Source: CAD feature listing. Evaluate the final solid. Frame: model axes, mm. Face numbers are marked on the shaded views. Coordinates: 2 decimals unless noted, no trailing zeros. Write each loop counter-clockwise with the first axis right and the second up, starting at its lowest first coordinate (ties: lowest second). Pieces come first, ordered by that corner, then holes. Notation, with made-up numbers: M 17.25,-23 L 46.25,-23 A27 cw 46.25,-7 Z; hole C -40,37 d2. An arc over 180 degrees is marked long. Answer as CSV lines item,"result". Start each with the question number.
1. Line query: probe 1 along Y at (x, z) = (14.4, 1.15) (3 decimals); probe 2 along X at (y, z) = (6.35, 0.2); probe 3 along Y at (x, z) = (25, 0.5). Output: solid intervals per line, ascending. Write a range as [from, to].
2. Section A-A on y = 6.35. Return the cut outline in (x, z) (1 decimal), plus the area to 3 significant figures.
3. Section C-C on x = 36.4. Return the cut outline in (y, z) (3 decimals), plus the area to 3 significant figures.
4. Section B-B on x = 25.4. Return the cut outline in (y, z) (3 decimals), plus the area to 3 significant figures.
5. Section D-D on y = 40. Return the cut outline in (x, z) (3 decimals), plus the area to 3 significant figures.
6. Mould query, pull axis X, two halves, no side actions, for the marked faces 1, 2 and 3. Classes: pulls with the +X half, pulls with the -X half, needs draft (parallel to the pull), parting line crosses it, or undercut.
7. Contact query for a flat-ended pin moving along its axis: pin 1 Ø12 at (x, y) = (19.5, 27.5) entering from -Z. Output: stop coordinate, or through.
Solid Edge part; units mm, degrees
sketch "Sketch1" plane through (0, 0, 0) normal (0, 0, 1) x (1, 0, 0)
  line L0 (0, 0) -> (50.8, 0)
  line L1 (50.8, 0) -> (50.8, 63.5)
  line L2 (50.8, 63.5) -> (0, 63.5)
  line L3 (0, 63.5) -> (0, 0)
extrude "Protrusion1" add sketch "Sketch1" along normal blind 3.175
hole "Hole_1" at (42.8625, 6.35, 3.175) direction (0, 0, -1) diameter 4.826 end up to next countersink diameter 9.525 countersink angle 82
hole "Hole1" at (7.9375, 6.35, 3.175) direction (0, 0, -1) diameter 4.826 end up to next countersink diameter 9.525 countersink angle 82
hole "Hole_2" at (25.4, 34.925, 3.175) direction (0, 0, -1) diameter 12.7 end up to next
chamfer "Chamfer_1" distance 6.35 angle 45 2 edges at (0, 63.5, 1.5875) (50.8, 63.5, 1.5875)
hole "Hole_4" at (36.4, 46.925, 3.175) direction (0, 0, -1) diameter 3.5 end up to next countersink diameter 6 countersink angle 82
hole "Hole2" at (36.4, 25.925, 3.175) direction (0, 0, -1) diameter 3.5 end up to next countersink diameter 6 countersink angle 82
hole "Hole3" at (14.4, 25.925, 3.175) direction (0, 0, -1) diameter 3.5 end up to next countersink diameter 6 countersink angle 82
hole "Hole4" at (14.4, 46.925, 3.175) direction (0, 0, -1) diameter 3.5 end up to next countersink diameter 6 countersink angle 82
properties part number "CHAS-04" material "Aluminum, 1060"
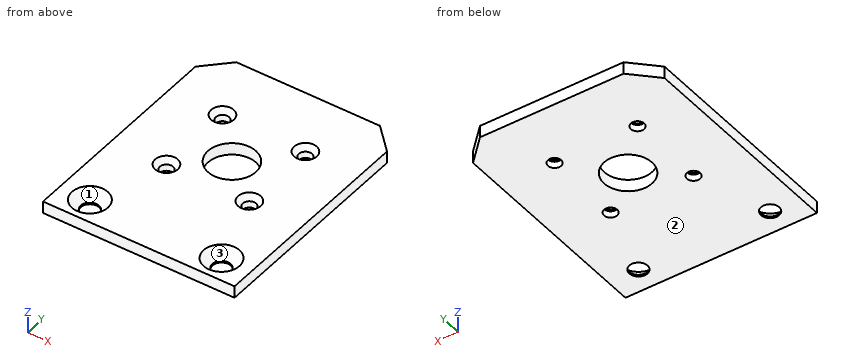
Values:
1,probe 1,"[0, 24.175], [27.675, 45.175], [48.675, 63.5]"
1,probe 2,"[0, 5.52], [10.35, 40.45], [45.28, 50.8]"
1,probe 3,"[0, 28.59], [41.26, 63.5]"
2,outline,"M 0,0 L 5.5,0 L 5.5,0.5 L 3.2,3.2 L 0,3.2 Z; M 10.4,0 L 40.4,0 L 40.4,0.5 L 38.1,3.2 L 12.7,3.2 L 10.4,0.5 Z; M 45.3,0 L 50.8,0 L 50.8,3.2 L 47.6,3.2 L 45.3,0.5 Z"
2,area,"118 mm²"
3,outline,"M 0,0 L 24.175,0 L 24.175,1.737 L 22.925,3.175 L 0,3.175 Z; M 27.675,0 L 45.175,0 L 45.175,1.737 L 43.925,3.175 L 28.925,3.175 L 27.675,1.737 Z; M 48.675,0 L 63.5,0 L 63.5,3.175 L 49.925,3.175 L 48.675,1.737 Z"
3,area,"176 mm²"
4,outline,"M 0,0 L 28.575,0 L 28.575,3.175 L 0,3.175 Z; M 41.275,0 L 63.5,0 L 63.5,3.175 L 41.275,3.175 Z"
4,area,"161 mm²"
5,outline,"M 0,0 L 21.583,0 L 21.583,3.175 L 0,3.175 Z; M 29.217,0 L 50.8,0 L 50.8,3.175 L 29.217,3.175 Z"
5,area,"137 mm²"
6,face 1,"undercut"
6,face 2,"needs draft"
6,face 3,"undercut"
7,pin 1,"z = 0"
